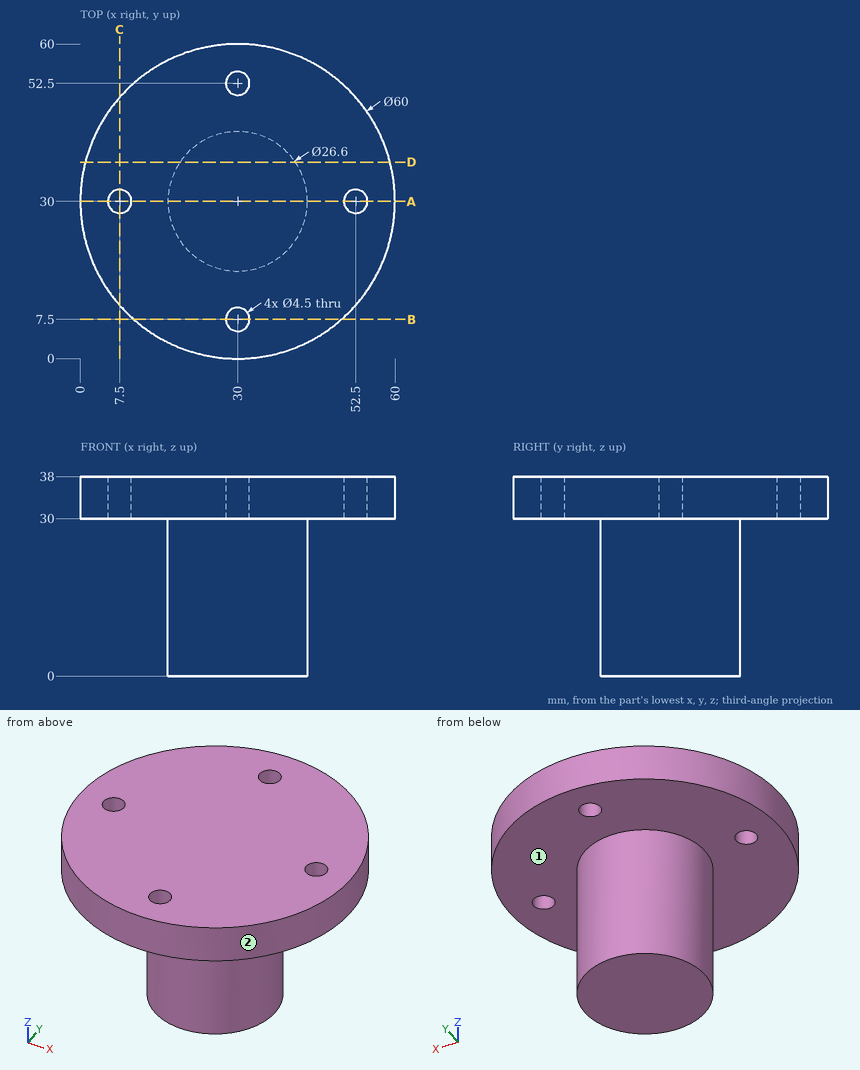
Answer from the drawing. Dimensions are ordinates in mm from the lowest x, y and z of the part. A direction names the side the tool comes from. Coordinates: 2 decimals unless noted, no trailing zeros. Write each loop counter-clockwise with the first axis right and the second up, starting at its lowest first coordinate (ties: lowest second). Pieces come first, ordered by that corner, then holes. Notation, with made-up numbers: (45.5, 44) - (89.5, 44) arc R16 ccw to (89.5, 50) - close; hole circle Ø7 at (24, 84.25). An arc over 180 degrees is marked (long way). Return JSON: item names as keys, results as strings.
1. The part is cut by section A-A on y = 30. Determine the outline of the cut face in (x, z), then the cut area to 3 significant figures.
Final values:
{"outline": "(0, 30) - (5.25, 30) - (5.25, 38) - (0, 38) - close; (9.75, 30) - (16.7, 30) - (16.7, 0) - (43.3, 0) - (43.3, 30) - (50.25, 30) - (50.25, 38) - (9.75, 38) - close; (54.75, 30) - (60, 30) - (60, 38) - (54.75, 38) - close", "area": "1,210 mm^2"}
2. The part is cut by section D-D on y = 37.5. Determine the outline of the cut face in (x, z), then the cut area to 3 significant figures.
Final values:
{"outline": "(0.95, 30) - (19.02, 30) - (19.02, 0) - (40.98, 0) - (40.98, 30) - (59.05, 30) - (59.05, 38) - (0.95, 38) - close", "area": "1,120 mm^2"}
3. Each of these flat-tipped pins is pushed along its axis until it touches: pin 1 Ø6 at (x, z) = (19.5, 28) entering from +Y; pin 2 Ø1 at (y, z) = (16, 33.5) entering from -X; pin 3 Ø3 at (x, y) = (34.5, 49) entering from -Z. Where does it stop, or does it pass through?
Final values:
{"pin 1": "y = 58.84", "pin 2": "x = 3.21", "pin 3": "z = 30"}
4. Consider line 1 along Y through (x, z) = (30, 36.5); line 2 along Y through (x, z) = (52.5, 33); line 3 along X through (y, z) = (7, 34). Determine where each line is inside the solid, lowest interval first.
Final values:
{"line 1": "0 to 5.25, 9.75 to 50.25, 54.75 to 60", "line 2": "10.16 to 27.75, 32.25 to 49.84", "line 3": "10.74 to 27.81, 32.19 to 49.26"}
5. Which of the six approach directions +Z, -Z, +X, -X, +Y, -Y give full straight-line access (tool end or side, diameter ignored) to the marked faces 1 and 2?
Final values:
{"face 1": "-Z", "face 2": "+Z, -Z"}
6. The part is cut by section B-B on y = 7.5. Determine the outline of the cut face in (x, z).
Final values:
{"outline": "(10.16, 30) - (27.75, 30) - (27.75, 38) - (10.16, 38) - close; (32.25, 30) - (49.84, 30) - (49.84, 38) - (32.25, 38) - close"}
